Input: part model. Units: mm. Frame: model coordinates. Face numbers are marked on the shaded views. A direction names the side the tool comes from. Coordinates: 2 decimals unless noted, no trailing zeros. Write each loop counter-clockwise with the first axis right and the second up, starting at its lowest first coordinate (ties: lowest second). Pieces come first, ordered by that corner, then holes. Notation, with made-up numbers: (22, 79.25) - (74, 79.25) arc R18 cw to (74, 85.25) - close; hole circle Ø10 at (58.25, 29). An arc over 180 degrees is marked (long way). Use CSV: the item, a comma, the result in double quotes.
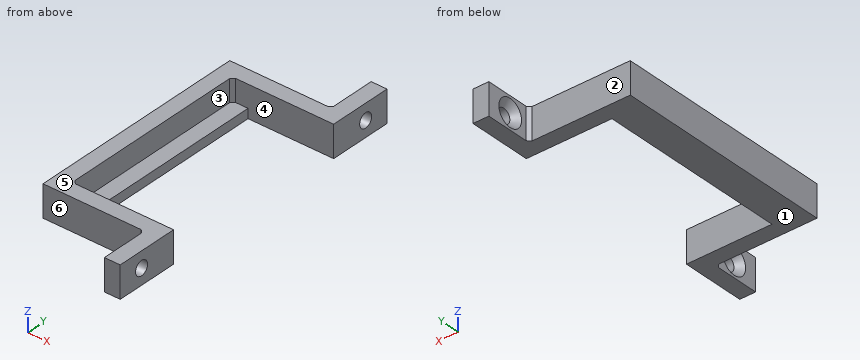
```python
from build123d import *

# Parameters (mm, degrees)
F1_DEPTH       = 10
F2_SIZE        = 1
F5_D           = 4.5
F5_CSINK_D     = 8.5
F5_CSINK_ANGLE = 90
F6_DEPTH       = 3


with BuildPart() as f1:
    # F0 (on Top) → F1 (new body)
    with BuildSketch(Plane.XY):
        Polygon((0, -30), (0, 0), (0, 30), (5, 30), (32, 30), (32, 50), (27, 50), (27, 35), (-5, 35), (-5, 0), (-5, -35), (27, -35), (27, -50), (32, -50), (32, -30), (5, -30), align=None)
    extrude(amount=F1_DEPTH)

    # F2
    f2_edges = [f1.edges().sort_by_distance(p)[0] for p in [
        (0, -30, 5),
        (27, -35, 5),
        (0, 30, 5),
        (27, 35, 5),
    ]]
    chamfer(f2_edges, length=F2_SIZE)

    # F5 (through all)
    with Locations(Plane(origin=(27, 0, 0), x_dir=(0, -1, 0), z_dir=(-1, 0, 0))):
        with Locations((42, 5), (-42, 5)):
            CounterSinkHole(F5_D / 2, F5_CSINK_D / 2, counter_sink_angle=F5_CSINK_ANGLE)

    # F0 (on Top) → F6 (join)
    with BuildSketch(Plane.XY):
        Polygon((0, 30), (0, 0), (0, -30), (5, -30), (5, 30), align=None)
    extrude(amount=F6_DEPTH)


solid = f1.part
```
(1) Reachability of the marked faces 5 and 6 from +Z, -Z, +X, -X, +Y, -Y: full face, straight path, thin tool, end or side. Return the list, or none.
Check values:
face 5,"+Z, +X, -X, +Y, -Y"
face 6,"+Z, -Z, -X, -Y"
(2) Draft query along Y for the marked faces 1, 2, 3 and 4. Return one class per face: pulls with the +Y half, pulls with the -Y half, needs draft (parallel to the pull), parting line crosses it, or undercut.
Check values:
face 1,"needs draft"
face 2,"pulls with the +Y half"
face 3,"undercut"
face 4,"undercut"
(3) Pin query (flat end, axial travel): pin 1 Ø5 at (y, z) = (42, 5) entering from -X; pin 2 Ø3.5 at (y, z) = (-7.5, 1.5) entering from +X; pin 3 Ø4 at (y, z) = (-42, 5) entering from -X; pin 4 Ø3 at (x, z) = (9.5, 4.5) entering from -Y. Return the tip coordinate at first contact, or that it passes through.
Check values:
pin 1,"x = 28.75"
pin 2,"x = 5"
pin 3,"through"
pin 4,"y = -35"
(4) Cut plane A-A on x = 8.5. Return loops of the section in (y, z).
Check values:
outline,"(-35, 0) - (-30, 0) - (-30, 10) - (-35, 10) - close; (30, 0) - (35, 0) - (35, 10) - (30, 10) - close"
(5) Cut plane D-D on y = 5. Return loops of the section in (x, z), and give its area (3 significant figures).
Check values:
outline,"(-5, 0) - (5, 0) - (5, 3) - (0, 3) - (0, 10) - (-5, 10) - close"
area,"65.0 mm^2"
(6) Cut plane C-C on y = -42. Return loops of the section in (x, z), and give its area (3 significant figures).
Check values:
outline,"(27, 0) - (32, 0) - (32, 2.75) - (29, 2.75) - (27, 0.75) - close; (27, 9.25) - (29, 7.25) - (32, 7.25) - (32, 10) - (27, 10) - close"
area,"23.5 mm^2"
(7) Ray query, probe 1 along Y at (x, z) = (30.35, 5); probe 2 along Z at (x, y) = (30.3, -42); probe 3 along Y at (x, z) = (18, 3). Return the intervals inside material, ascending. Write a range as from..to.
Check values:
probe 1,"-50..-44.25, -39.75..-30, 30..39.75, 44.25..50"
probe 2,"0..2.75, 7.25..10"
probe 3,"-35..-30, 30..35"
(8) Cut plane B-B on z = 5. Return loops of the section in (x, y).
Check values:
outline,"(-5, -35) - (26, -35) - (27, -36) - (27, -37.75) - (29, -39.75) - (32, -39.75) - (32, -30) - (1, -30) - (0, -29) - (0, 29) - (1, 30) - (32, 30) - (32, 39.75) - (29, 39.75) - (27, 37.75) - (27, 36) - (26, 35) - (-5, 35) - close; (27, -50) - (32, -50) - (32, -44.25) - (29, -44.25) - (27, -46.25) - close; (27, 46.25) - (29, 44.25) - (32, 44.25) - (32, 50) - (27, 50) - close"
